Work out the finished part from the listing and answer in its coordinate system (mm). Face numbers are marked on the shaded views. A direction names the side the tool comes from. Give positions to 0.01 mm unless a question says otherwise; leave off trailing zeros. Loops run counter-clockwise (first coordinate to the right, second up) from the corner with the lowest first, then second, coordinate; pieces in that order, holes last. Notation, with made-up numbers: M 38,-12.75 L 85,-12.75 A23 ccw 85,26.25 Z; hole C 75,11.25 d7. An arc over 180 degrees is marked long. Use a Markdown table: item, result.
```python
from build123d import *

# Parameters (mm, degrees)
PAD010_DEPTH    = 10
POCKET004_DEPTH = 2
SKETCH021_R     = 2.2
POCKET005_DEPTH = 23.001
CHAMFER004_SIZE = 2
PAD016_DEPTH    = 2


with BuildPart() as part:
    # Sketch019 → Pad010 (new body)
    with BuildSketch(Plane.YZ):
        with BuildLine():
            ThreePointArc((-13.416408, -1.5), (13.5, 0), (-13.416408, 1.5))
            Line((-13.416408, 1.5), (-26.613248, 1.5))
            Line((-26.613248, 5.5), (-26.613248, 1.5))
            Line((-16.613248, 5.5), (-26.613248, 5.5))
            ThreePointArc((-16.613248, -5.5), (17.5, 0), (-16.613248, 5.5))
            Line((-16.613248, -5.5), (-26.613248, -5.5))
            Line((-26.613248, -1.5), (-26.613248, -5.5))
            Line((-13.416408, -1.5), (-26.613248, -1.5))
        make_face()
    extrude(amount=PAD010_DEPTH)

    # Sketch020 (on DatumPlane) → Pocket004 (cut)
    with BuildSketch(Plane.XY.offset(-5.5)):
        Polygon((7.049593, -25.163248), (9.099187, -21.613248), (7.049593, -18.063248), (2.950407, -18.063248), (0.900813, -21.613248), (2.950407, -25.163248), align=None)
    extrude(amount=POCKET004_DEPTH, mode=Mode.SUBTRACT)

    # Sketch021 (on DatumPlane) → Pocket005 (cut, through all)
    with BuildSketch(Plane.XY.offset(5.5)):
        with Locations((5, -21.613248)):
            Circle(SKETCH021_R)
    extrude(amount=-POCKET005_DEPTH, mode=Mode.SUBTRACT)

    # Chamfer004
    chamfer004_edges = [part.edges().sort_by_distance(p)[0] for p in [
        (10, -26.613248, 3.5),
        (10, -26.613248, -3.5),
        (0, -26.613248, 3.5),
        (0, -26.613248, -3.5),
    ]]
    chamfer(chamfer004_edges, length=CHAMFER004_SIZE)

    # Sketch028 → Pad016 (join)
    with BuildSketch(Plane.YZ):
        with BuildLine():
            ThreePointArc((8, -17.5), (25.5, 0), (8, 17.5))
            Line((0, 17.5), (8, 17.5))
            ThreePointArc((0, -17.5), (17.5, 0), (0, 17.5))
            Line((0, -17.5), (8, -17.5))
        make_face()
    extrude(amount=PAD016_DEPTH)


solid = part.part
```
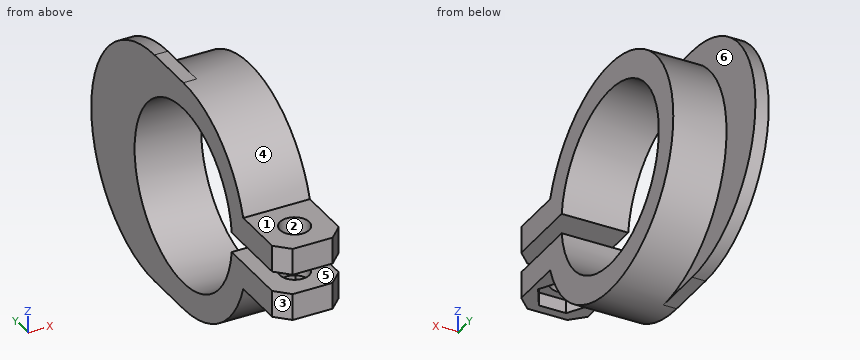
(1) Consider probe 1 along Z at (x, y) = (2, -17.5); probe 2 along Y at (x, z) = (5, -2.25); probe 3 along Y at (x, z) = (5, -2.6). Determine where each line is inside the solid, lowest interval first. Write a range as [from, to].
Entries:
| item | result |
|---|---|
| probe 1 | z = [-5.5, -1.5], [1.5, 5.5] |
| probe 2 | y = [-26.61, -23.81], [-19.41, -13.31], [13.31, 17.35] |
| probe 3 | y = [-26.61, -23.81], [-19.41, -13.25], [13.25, 17.31] |
(2) A cutting plane is placed at C-C (y = -5.5). Write down the section's boundary in (x, z), and give its area (3 significant figures).
Entries:
| item | result |
|---|---|
| outline | M 0,-16.61 L 10,-16.61 L 10,-12.33 L 0,-12.33 Z; M 0,12.33 L 10,12.33 L 10,16.61 L 0,16.61 Z |
| area | 85.7 mm² |
(3) A cutting plane is placed at A-A (x = 5). Write down the section's boundary in (y, z).
Entries:
| item | result |
|---|---|
| outline | M -26.61,-5.5 L -25.16,-5.5 L -25.16,-3.5 L -23.81,-3.5 L -23.81,-1.5 L -26.61,-1.5 Z; M -26.61,1.5 L -23.81,1.5 L -23.81,5.5 L -26.61,5.5 Z; M -19.41,-3.5 L -18.06,-3.5 L -18.06,-5.5 L -16.61,-5.5 A17.5 ccw long -16.61,5.5 L -19.41,5.5 L -19.41,1.5 L -13.42,1.5 A13.5 cw long -13.42,-1.5 L -19.41,-1.5 Z |
(4) A cutting plane is placed at D-D (z = -11.5). Write down the section's boundary in (x, y).
Entries:
| item | result |
|---|---|
| outline | M 0,-13.19 L 10,-13.19 L 10,-7.07 L 0,-7.07 Z; M 0,7.07 L 10,7.07 L 10,13.19 L 2,13.19 L 2,21.19 L 0,21.19 Z |
(5) Given P1, Ø20.5, axis at y = 9.5, z = 0, coming from the +X side; P2, Ø1, axis at x = 6, y = -7.5, coming from the -Z side; P3, Ø3.5, axis at x = 6.5, y = -22, coming from the -Z side; P4, Ø5, axis at x = 3, y = -20.5, coming from the +Z side, each flat-ended and moving along its own axis, determine where each tip first touches the part or whether it passes through.
Entries:
| item | result |
|---|---|
| P1 | stops at x = 10 |
| P2 | stops at z = -16.04 |
| P3 | stops at z = -3.5 |
| P4 | stops at z = 5.5 |
(6) A cutting plane is placed at B-B (z = 2.5). Write down the section's boundary in (x, y).
Entries:
| item | result |
|---|---|
| outline | M 0,-24.61 L 2,-26.61 L 8,-26.61 L 10,-24.61 L 10,-13.27 L 0,-13.27 Z; M 0,13.27 L 10,13.27 L 10,17.32 L 2,17.32 L 2,25.32 L 0,25.32 Z; hole C 5,-21.61 d4.4 |
(7) Which of the six approach directions +Z, -Z, +X, -X, +Y, -Y give full straight-line access (tool end or side, diameter ignored) to the marked faces 4, 5 and 6?
Entries:
| item | result |
|---|---|
| face 4 | +X |
| face 5 | +X, -X, -Y |
| face 6 | +X, +Y |
(8) The mould has two halves that part along Y. Classify the marked faces 1, 2 and 3: released by +Y, released by -Y, zero draft, split by the parting line, or undercut.
Entries:
| item | result |
|---|---|
| face 1 | zero draft |
| face 2 | undercut |
| face 3 | released by -Y |
